Source: CAD feature listing. Evaluate the final solid. Frame: model axes, mm. Face numbers are marked on the shaded views. A direction names the side the tool comes from. Round coordinates to 2 decimals unless told otherwise and drop trailing zeros. Order: outer loops, then holes, each group sorted by start corner. A loop starts at its lowest first (then second) coordinate and runs counter-clockwise, first axis right, second up. Notation, with made-up numbers: (51, 2) - (86, 2) arc R13 ccw to (86, 6) - close; hole circle Ø6 at (84, 65). An arc over 180 degrees is marked (long way). Put each result on its own line as item: value. Start each with the question number.
1) Line query: probe 1 along Z at (x, y) = (8, 93.5); probe 2 along X at (y, z) = (167, 734); probe 3 along Y at (x, z) = (1.9, 808.14). Output: solid intervals per line, ascending. Write a range as [from, to].
2) Contact query for flat-ended pins moving along their axis: P1, Ø18.5, axis at y = 100, z = 594, coming from the -X side; P2, Ø20, axis at y = 158, z = 449, coming from the +X side; P3, Ø9, axis at y = 170, z = 808.14, coming from the -X side. Output: stop coordinate, or through.
3) Mould query, pull axis Y, two halves, no side actions, for the marked faces 3 and 4. Classes: +Y half, -Y half, draft (parallel to the pull), parting line (faces both ways), or undercut.
4) Section B-B on z = 673.5. Output: boundary loops of the cut face in (x, y).
5) Access query for the marked faces 1 and 2. Directions: +Z, -Z, +X, -X, +Y, -Y. A direction counts if a zero-diameter tool reaches every point of the face in a straight line with its end or side. Return the directions, or none.
6) Section A-A on z = 130. Output: boundary loops of the cut face in (x, y).
```python
from build123d import *

# Parameters (mm, degrees)
EXTRUDE_1_DEPTH             = 824
FILLET_1_R                  = 4
FILLET_2_R                  = 2
HOLE_WIZARD_16_0_16_1_D     = 16
HOLE_WIZARD_16_0_16_1_DEPTH = 24.5
HOLE_WIZARD_16_0_16_1_TIP   = 4.806884952
HOLE_WIZARD_10_0_10_1_D     = 10


with BuildPart() as part:
    # 草图1 → 凸台-拉伸1 (new body)
    with BuildSketch(Plane.XY):
        Polygon((0, 0), (0, 67.749635555), (7, 76.091910703), (7, 123.908089297), (0, 132.250364445), (0, 200), (3, 200), (3, 133.342275148), (10, 125), (10, 75), (3, 66.657724852), (3, 0), align=None)
    extrude(amount=EXTRUDE_1_DEPTH)

    # 圆角1
    fillet_1_edges = [part.edges().sort_by_distance(p)[0] for p in [
        (0, 67.749635555, 412),
        (0, 132.250364445, 412),
        (10, 125, 412),
        (10, 75, 412),
    ]]
    fillet(fillet_1_edges, radius=FILLET_1_R)

    # 圆角2
    fillet_2_edges = [part.edges().sort_by_distance(p)[0] for p in [
        (7, 76.091910703, 412),
        (7, 123.908089297, 412),
        (3, 133.342275148, 412),
        (3, 66.657724852, 412),
    ]]
    fillet(fillet_2_edges, radius=FILLET_2_R)

    # Ø16.0 (16) 直径孔1
    with Locations(Plane(origin=(10, 0, 0), x_dir=(0, 0, -1), z_dir=(1, 0, 0))):
        with Locations((-694, 100), (-130, 100), (-594, 100), (-230, 100)):
            Hole(HOLE_WIZARD_16_0_16_1_D / 2, depth=HOLE_WIZARD_16_0_16_1_DEPTH)
            with Locations((0, 0, -(HOLE_WIZARD_16_0_16_1_DEPTH + HOLE_WIZARD_16_0_16_1_TIP / 2))):  # 118° drill point
                Cone(0, HOLE_WIZARD_16_0_16_1_D / 2, HOLE_WIZARD_16_0_16_1_TIP, mode=Mode.SUBTRACT)

    # Ø10.0 (10) 直径孔1 (through all)
    with Locations(Plane.ZY):
        with Locations((8.14, 170), (8.14, 30), (808.14, 170), (808.14, 30)):
            Hole(HOLE_WIZARD_10_0_10_1_D / 2)


solid = part.part
```
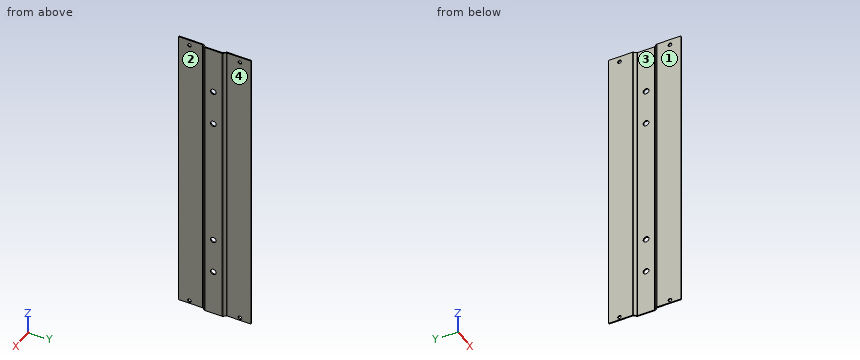
Answer sheet:
1. probe 1: [0, 125.34], [134.66, 225.34], [234.66, 589.34], [598.66, 689.34], [698.66, 824]
1. probe 2: [0, 3]
1. probe 3: [0, 25], [35, 70.01], [129.99, 165], [175, 200]
2. P1: x = 7
2. P2: x = 3
2. P3: through
3. face 3: undercut
3. face 4: draft
4. outline: (0, 0) - (3, 0) - (3, 65.93) arc R2 cw to (3.47, 67.22) - (9.06, 73.88) arc R4 ccw to (10, 76.46) - (10, 123.54) arc R4 ccw to (9.06, 126.12) - (3.47, 132.78) arc R2 cw to (3, 134.07) - (3, 200) - (0, 200) - (0, 133.71) arc R4 ccw to (0.94, 131.14) - (6.53, 124.47) arc R2 cw to (7, 123.18) - (7, 76.82) arc R2 cw to (6.53, 75.53) - (0.94, 68.86) arc R4 ccw to (0, 66.29) - close
5. face 1: +Z, -Z, -X, +Y, -Y
5. face 2: +Z, -Z, +X, -Y
6. outline: (0, 0) - (3, 0) - (3, 65.93) arc R2 cw to (3.47, 67.22) - (9.06, 73.88) arc R4 ccw to (10, 76.46) - (10, 92) - (7, 92) - (7, 76.82) arc R2 cw to (6.53, 75.53) - (0.94, 68.86) arc R4 ccw to (0, 66.29) - close; (0, 133.71) arc R4 ccw to (0.94, 131.14) - (6.53, 124.47) arc R2 cw to (7, 123.18) - (7, 108) - (10, 108) - (10, 123.54) arc R4 ccw to (9.06, 126.12) - (3.47, 132.78) arc R2 cw to (3, 134.07) - (3, 200) - (0, 200) - close
